Source: CAD feature listing. Evaluate the final solid. Frame: model axes, mm. A direction names the side the tool comes from. Round coordinates to 2 decimals unless told otherwise and drop trailing zeros. Write each loop counter-clockwise with the first axis right and the second up, starting at its lowest first coordinate (ties: lowest second). Pieces come first, ordered by that corner, then holes. Notation, with made-up numbers: M -24,32 L 3,32 A18 ccw 3,37 Z; hole C 46,85 d11. An arc over 180 degrees is marked long. Use a Markdown table: item, result.
```python
from build123d import *

# Parameters (mm, degrees)
F0_R      = 6
F1_DEPTH  = 20
F2_W      = 14.4337567297
F2_H      = 30
F3_DEPTH  = 20
F4_R      = 4.5
F5_DEPTH  = 21.6516350946
F7_DEPTH  = 25.4
F8_W      = 4.4337567297
F8_H      = 40
F9_DEPTH  = 25.4
F10_W     = 14.4337567297
F10_H     = 30
F11_DEPTH = 20
F12_R     = 4.5
F13_DEPTH = 25.4
F15_DEPTH = 25.4
F16_W     = 4.4337567297
F16_H     = 40
F17_DEPTH = 25.4


with BuildPart() as f1:
    # F0 (on Front) → F1 (new body, symmetric)
    with BuildSketch(Plane.XZ):
        Polygon((7.2168783649, 12.5), (-7.2168783649, 12.5), (-14.4337567297, 0), (-7.2168783649, -12.5), (7.2168783649, -12.5), (14.4337567297, 0), align=None)
        Circle(F0_R, mode=Mode.SUBTRACT)
    extrude(amount=F1_DEPTH, both=True)

    # F2 (on face) → F3 (join)
    with BuildSketch(Plane.XY.offset(12.5)):
        Rectangle(F2_W, F2_H)
    extrude(amount=F3_DEPTH)

    # F4 (on face) → F5 (cut, through all)
    with BuildSketch(Plane(origin=(-7.2168783649, 0, 0), x_dir=(0, -1, 0), z_dir=(-1, 0, 0))):
        with Locations((0, 22.5)):
            Circle(F4_R)
    extrude(amount=-F5_DEPTH, mode=Mode.SUBTRACT)

    # F6 (on face) → F7 (cut)
    with BuildSketch(Plane(origin=(-7.2168783649, 0, 0), x_dir=(0, -1, 0), z_dir=(-1, 0, 0))):
        with BuildLine():
            Line((-15, 32.5), (-15, 12.5))
            Line((-15, 12.5), (-9.2307692308, 26.3461538462))
            ThreePointArc((-9.2307692308, 26.3461538462), (-5.5470019623, 30.8205029434), (0, 32.5))
            Line((0, 32.5), (-15, 32.5))
        make_face()
        with BuildLine():
            Line((9.2307692308, 26.3461538462), (15, 12.5))
            Line((15, 12.5), (15, 32.5))
            Line((15, 32.5), (0, 32.5))
            ThreePointArc((0, 32.5), (5.5470019623, 30.8205029434), (9.2307692308, 26.3461538462))
        make_face()
    extrude(amount=-F7_DEPTH, mode=Mode.SUBTRACT)

    # F8 (on face) → F9 (cut)
    with BuildSketch(Plane.XY.offset(12.5)):
        Rectangle(F8_W, F8_H)
    extrude(amount=F9_DEPTH, mode=Mode.SUBTRACT)

    # F10 (on face) → F11 (join)
    with BuildSketch(Plane(origin=(0, 0, -12.5), x_dir=(1, 0, 0), z_dir=(0, 0, -1))):
        Rectangle(F10_W, F10_H)
    extrude(amount=F11_DEPTH)

    # F12 (on face) → F13 (cut)
    with BuildSketch(Plane.YZ.offset(7.2168783649)):
        with Locations((0, -22.5)):
            Circle(F12_R)
    extrude(amount=-F13_DEPTH, mode=Mode.SUBTRACT)

    # F14 (on face) → F15 (cut)
    with BuildSketch(Plane.YZ.offset(7.2168783649)):
        with BuildLine():
            Line((15, -32.5), (15, -12.5))
            Line((15, -12.5), (9.2307692308, -26.3461538462))
            ThreePointArc((9.2307692308, -26.3461538462), (5.5470019443, -30.8205029554), (-4.32e-08, -32.5))
            Line((-4.32e-08, -32.5), (15, -32.5))
        make_face()
        with BuildLine():
            Line((-9.2307692308, -26.3461538462), (-15, -12.5))
            Line((-15, -12.5), (-15, -32.5))
            Line((-15, -32.5), (-4.32e-08, -32.5))
            ThreePointArc((-4.32e-08, -32.5), (-5.5470019802, -30.8205029314), (-9.2307692308, -26.3461538462))
        make_face()
    extrude(amount=-F15_DEPTH, mode=Mode.SUBTRACT)

    # F16 (on face) → F17 (cut)
    with BuildSketch(Plane(origin=(0, 0, -12.5), x_dir=(1, 0, 0), z_dir=(0, 0, -1))):
        Rectangle(F16_W, F16_H)
    extrude(amount=F17_DEPTH, mode=Mode.SUBTRACT)


solid = f1.part
```
Q1. Section D-D on x = 5. Return loops of the section in (y, z), plus the area to 3 significant figures.
Results are:
| item | result |
|---|---|
| outline | M -20,-12.5 L -15,-12.5 L -9.23,-26.35 A10 ccw 9.23,-26.35 L 15,-12.5 L 20,-12.5 L 20,-3.32 L -20,-3.32 Z; M -20,3.32 L 20,3.32 L 20,12.5 L 15,12.5 L 9.23,26.35 A10 ccw -9.23,26.35 L -15,12.5 L -20,12.5 Z; hole C 0,-22.5 d9; hole C 0,22.5 d9 |
| area | 1,440 mm^2 |
Q2. Section C-C on z = 28.5. Return loops of the section in (x, y), plus the area to 3 significant figures.
Results are:
| item | result |
|---|---|
| outline | M -7.22,-8 L -2.22,-8 L -2.22,8 L -7.22,8 Z; M 2.22,-8 L 7.22,-8 L 7.22,8 L 2.22,8 Z |
| area | 160 mm^2 |
Q3. Line query: L1, parallel to X at y = 0, z = 13.5; L2, parallel to Z at x = -1.75, y = 11; L3, parallel to Y at x = -4.5, z = -19.5. Output: solid intervals per line, ascending.
Results are:
| item | result |
|---|---|
| L1 | -7.22 to -2.22, 2.22 to 7.22 |
| L2 | -12.5 to -5.74, 5.74 to 12.5 |
| L3 | -12.08 to -3.35, 3.35 to 12.08 |
Q4. Section A-A on x = 0. Return loops of the section in (y, z), plus the area to 3 significant figures.
Results are:
| item | result |
|---|---|
| outline | M -20,-12.5 L 20,-12.5 L 20,-6 L -20,-6 Z; M -20,6 L 20,6 L 20,12.5 L -20,12.5 Z |
| area | 520 mm^2 |
Q5. Section B-B on y = 10. Return loops of the section in (x, z), plus the area to 3 significant figures.
Results are:
| item | result |
|---|---|
| outline | M -14.43,0 L -7.22,-12.5 L -7.22,-24.5 L -2.22,-24.5 L -2.22,-12.5 L 2.22,-12.5 L 2.22,-24.5 L 7.22,-24.5 L 7.22,-12.5 L 14.43,0 L 7.22,12.5 L 7.22,24.5 L 2.22,24.5 L 2.22,12.5 L -2.22,12.5 L -2.22,24.5 L -7.22,24.5 L -7.22,12.5 Z; hole C 0,0 d12 |
| area | 668 mm^2 |
Q6. First-contact query: pin 1 Ø8 at (y, z) = (0, -22.5) entering from +X; pin 2 Ø6 at (y, z) = (-2.5, 25) entering from -X; pin 3 Ø6 at (y, z) = (1, 27) entering from +X; pin 4 Ø12 at (y, z) = (-7, 12.5) entering from -X. Flat tips, straight axial feed; report the tip coordinate or a pass-through.
Results are:
| item | result |
|---|---|
| pin 1 | through |
| pin 2 | x = -7.22 |
| pin 3 | x = 7.22 |
| pin 4 | x = -10.68 |
Q7. Mould query, pull axis Z, two halves, no side actions, for faces 1 (the flat face through (7.217, -3, -18)), 2 (the cylindrical face through (4.75, -0.59, -18.04)), 3 (the flat face through (-4.682, 12.156, -19.326)). Classes: +Z half, -Z half, draft (parallel to the pull), parting line (faces both ways), or undercut.
Results are:
| item | result |
|---|---|
| face 1 | draft |
| face 2 | undercut |
| face 3 | -Z half |
Q8. Reachability of faces 4 (the flat face through (0, 0, 12.5)), 5 (the flat face through (7.217, 3, 18)), 6 (the flat face through (-2.217, 3, 18)), 7 (the flat face through (0, 0, -12.5)) from +Z, -Z, +X, -X, +Y, -Y: full face, straight path, thin tool, end or side. Return the list, or none.
Results are:
| item | result |
|---|---|
| face 4 | +Z |
| face 5 | +Z, +X, +Y, -Y |
| face 6 | +Z, +Y, -Y |
| face 7 | -Z |
